The model under review builds one solid part; all positions refer to its coordinate system, in mm. Face numbers are marked on the shaded views. A direction names the side the tool comes from. Coordinates: 2 decimals unless noted, no trailing zeros. Order: outer loops, then holes, each group sorted by start corner. A loop starts at its lowest first (then second) coordinate and runs counter-clockwise, first axis right, second up. Notation, with made-up numbers: M -25,72 L -2,72 A24 ccw -2,110 Z; hole C 45.25,60.5 d4. An arc over 180 degrees is marked long. One line per item, written item: value.
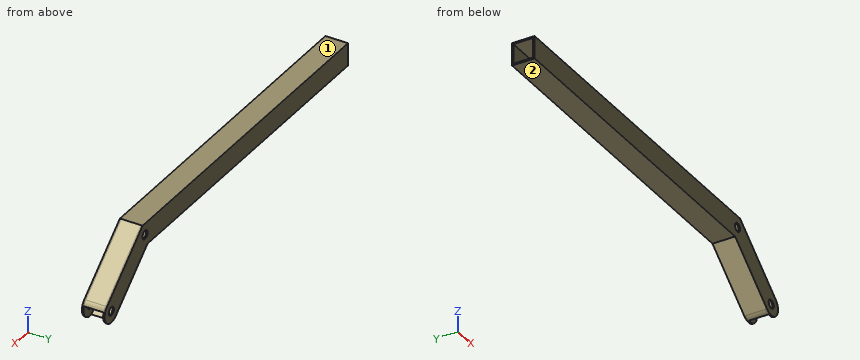
```python
from build123d import *

# Parameters (mm, degrees)
BOSS_EXTRUDE5_DEPTH = 1.5875
BOSS_EXTRUDE6_DEPTH = 22.225
BOSS_EXTRUDE7_DEPTH = 22.225
BOSS_EXTRUDE8_DEPTH = 1.5875
HOLE1_OUTLINE_R     = 4.826
HOLE1_DEPTH         = 25.4
HOLE2_OUTLINE_R     = 4.826
HOLE2_DEPTH         = 25.4


# Read off the part's stored shape, not the designer's step: Hole1, Hole2
with BuildPart() as part:
    # Sketch9 → Boss-Extrude5 (new body)
    with BuildSketch(Plane(origin=(0, 0, 0), x_dir=(1, 0, 0), z_dir=(0, 1, 0))):
        with BuildLine():
            Line((322.629578317, 36.567646265), (382.325566472, 86.658527908))
            ThreePointArc((382.325566472, 86.658527908), (400.217733608, 85.093166118), (398.652371818, 67.200998981))
            Line((398.652371818, 67.200998981), (331.874422413, 11.167646265))
            Line((331.874422413, 11.167646265), (-53.747999635, 11.167646265))
            Line((-53.747999635, 11.167646265), (-53.747999635, 36.567646265))
            Line((-53.747999635, 36.567646265), (322.629578317, 36.567646265))
        make_face()
    extrude(amount=BOSS_EXTRUDE5_DEPTH)

    # Sketch11 → Boss-Extrude6 (add)
    with BuildSketch(Plane(origin=(0, 1.5875, 0), x_dir=(1, 0, 0), z_dir=(0, 1, 0))):
        with BuildLine():
            Line((323.207381137, 34.980146265), (-53.747999635, 34.980146265))
            Line((-53.747999635, 34.980146265), (-53.747999635, 36.567646265))
            Line((-53.747999635, 36.567646265), (322.62957839, 36.567646265))
            Line((322.62957839, 36.567646265), (382.325566502, 86.658527872))
            ThreePointArc((382.325566502, 86.658527872), (385.016979631, 88.390449757), (388.055909658, 89.394522629))
            Line((388.055909658, 89.394522629), (323.207381137, 34.980146265))
        make_face()
    extrude(amount=BOSS_EXTRUDE6_DEPTH)

    # Sketch12 → Boss-Extrude7 (add)
    with BuildSketch(Plane(origin=(0, 1.5875, 0), x_dir=(1, 0, 0), z_dir=(0, 1, 0))):
        with BuildLine():
            Line((331.874422341, 13.239980337), (402.341864283, 72.369184881))
            ThreePointArc((402.341864283, 72.369184881), (400.825340873, 69.550778454), (398.652371788, 67.200999017))
            Line((398.652371788, 67.200999017), (331.874422341, 11.167646265))
            Line((331.874422341, 11.167646265), (-53.747999635, 11.167646265))
            Line((-53.747999635, 11.167646265), (-53.747999635, 12.755146265))
            Line((-53.747999635, 12.755146265), (330.542351676, 12.755146265))
            Line((330.542351676, 12.755146265), (330.85399701, 12.383741818))
            Line((330.85399701, 12.383741818), (331.296619594, 12.755146265))
            Line((331.296619594, 12.755146265), (331.874422341, 12.755146265))
            Line((331.874422341, 12.755146265), (331.874422341, 13.239980337))
        make_face()
    extrude(amount=BOSS_EXTRUDE7_DEPTH)

    # Sketch13 → Boss-Extrude8 (add)
    with BuildSketch(Plane(origin=(0, 23.8125, 0), x_dir=(1, 0, 0), z_dir=(0, 1, 0))):
        with BuildLine():
            Line((322.629578317, 36.567646265), (382.325566472, 86.658527908))
            ThreePointArc((382.325566472, 86.658527908), (400.217733608, 85.093166118), (398.652371818, 67.200998981))
            Line((398.652371818, 67.200998981), (331.874422413, 11.167646265))
            Line((331.874422413, 11.167646265), (-53.747999635, 11.167646265))
            Line((-53.747999635, 11.167646265), (-53.747999635, 36.567646265))
            Line((-53.747999635, 36.567646265), (322.629578317, 36.567646265))
        make_face()
    extrude(amount=BOSS_EXTRUDE8_DEPTH)

    # Hole1 outline → Hole1 (cut)
    with BuildSketch(Plane(origin=(0, 0, 0), x_dir=(1, 0, 0), z_dir=(0, 1, 0))):
        with Locations((327.252000365, 23.867646265)):
            Circle(HOLE1_OUTLINE_R)
    extrude(amount=HOLE1_DEPTH, mode=Mode.SUBTRACT)

    # Hole2 outline → Hole2 (cut)
    with BuildSketch(Plane(origin=(0, 0, 0), x_dir=(1, 0, 0), z_dir=(0, 1, 0))):
        with Locations((390.488969145, 76.929763445)):
            Circle(HOLE2_OUTLINE_R)
    extrude(amount=HOLE2_DEPTH, mode=Mode.SUBTRACT)


solid = part.part
```
(1) For L1, parallel to Z at x = 141.5, y = 15.5; L2, parallel to Y at x = 62.5, z = -23.5; L3, parallel to X at y = 7.5, z = -64.5, list the stretches that pass through material, from the lowest coordinate up.
Geometry results:
L1: z = -36.57 to -34.98, -12.76 to -11.17
L2: y = 0 to 1.59, 23.81 to 25.4
L3: x = 355.92 to 358.39, 392.96 to 395.43
(2) We need section C-C, the plane z = -60.5. State the section outline as (x, y) points.
Geometry results:
outline: M 351.15,0 L 390.67,0 L 390.67,25.4 L 351.15,25.4 Z; hole M 353.62,1.59 L 388.2,1.59 L 388.2,23.81 L 353.62,23.81 Z
(3) Tool access review of the marked faces 1 and 2: name each direction out of +Z, -Z, +X, -X, +Y, -Y from which nothing blocks a thin tool from reaching the whole face with its end or side.
Geometry results:
face 1: +Z, +X, -X, +Y, -Y
face 2: -Z, -X, +Y, -Y
(4) We need section A-A, the plane y = 19.5. State the section outline as (x, z) points.
Geometry results:
outline: M -53.75,-36.57 L 322.63,-36.57 L 382.33,-86.66 A12.7 ccw 388.06,-89.39 L 323.21,-34.98 L -53.75,-34.98 Z; M -53.75,-12.76 L 330.54,-12.76 L 330.85,-12.38 L 331.3,-12.76 L 331.87,-12.76 L 331.87,-13.24 L 402.34,-72.37 A12.7 ccw 398.65,-67.2 L 331.87,-11.17 L -53.75,-11.17 Z
(5) We need section D-D, the plane x = 358.5. State the section outline as (y, z) points, plus the area to 3 significant figures.
Geometry results:
outline: M 0,-66.67 L 25.4,-66.67 L 25.4,-33.51 L 0,-33.51 Z; hole M 1.59,-64.59 L 23.81,-64.59 L 23.81,-35.58 L 1.59,-35.58 Z
area: 197 mm2
(6) We need section B-B, the plane x = 242. State the section outline as (y, z) points.
Geometry results:
outline: M 0,-36.57 L 25.4,-36.57 L 25.4,-11.17 L 0,-11.17 Z; hole M 1.59,-34.98 L 23.81,-34.98 L 23.81,-12.76 L 1.59,-12.76 Z
(7) Insertion check: pin 1 Ø4 at (x, y) = (332.5, 20) entering from +Z; pin 2 Ø5 at (x, y) = (175, 5) entering from -Z; pin 3 Ø4 at (y, z) = (7, -34) entering from +X; pin 4 Ø3 at (x, y) = (350.5, 10) entering from +Z. Each pin has a flat end and moves straight along its axis. Give the tip position at first contact, or say it passes through.
Geometry results:
pin 1: stops at z = -11.17
pin 2: stops at z = -36.57
pin 3: stops at x = 361.47
pin 4: stops at z = -25.54
